```python
from build123d import *

# Parameters (mm, degrees)
SKETCH1_R           = 7.3
SKETCH1_R_2         = 2.4
BOSS_EXTRUDE1_DEPTH = 10
SKETCH2_R           = 8.8
SKETCH2_R_2         = 7.3
BOSS_EXTRUDE2_DEPTH = 3
SKETCH3_R           = 8.8
SKETCH3_R_2         = 2.4
BOSS_EXTRUDE3_DEPTH = 6
SKETCH4_R           = 4.2
SKETCH4_R_2         = 2.4
CUT_EXTRUDE1_DEPTH  = 43
BOSS_EXTRUDE4_REACH = 18
SKETCH5_R           = 7.5
SKETCH5_R_2         = 7.3
SKETCH6_R           = 4.2
SKETCH6_R_2         = 4.1
BOSS_EXTRUDE5_DEPTH = 16


with BuildPart() as part:
    # Sketch1 → Boss-Extrude1 (new body)
    with BuildSketch(Plane(origin=(0, 0, 0), x_dir=(1, 0, 0), z_dir=(0, 1, 0))):
        Circle(SKETCH1_R)
        Circle(SKETCH1_R_2, mode=Mode.SUBTRACT)
    extrude(amount=BOSS_EXTRUDE1_DEPTH)

    # Sketch2 → Boss-Extrude2 (add)
    with BuildSketch(Plane(origin=(0, 10, 0), x_dir=(1, 0, 0), z_dir=(0, 1, 0))):
        Circle(SKETCH2_R)
        Circle(SKETCH2_R_2, mode=Mode.SUBTRACT)
    extrude(amount=-BOSS_EXTRUDE2_DEPTH)

    # Sketch3 → Boss-Extrude3 (add)
    with BuildSketch(Plane(origin=(0, 10, 0), x_dir=(1, 0, 0), z_dir=(0, 1, 0))):
        Circle(SKETCH3_R)
        Circle(SKETCH3_R_2, mode=Mode.SUBTRACT)
    extrude(amount=BOSS_EXTRUDE3_DEPTH)

    # Sketch4 → Cut-Extrude1 (cut)
    with BuildSketch(Plane(origin=(0, 16, 0), x_dir=(1, 0, 0), z_dir=(0, 1, 0))):
        Circle(SKETCH4_R)
        Circle(SKETCH4_R_2, mode=Mode.SUBTRACT)
    extrude(amount=-CUT_EXTRUDE1_DEPTH, mode=Mode.SUBTRACT)

    # Sketch5 → Boss-Extrude4 (add, up to next)
    with BuildSketch(Plane.XZ, mode=Mode.PRIVATE) as boss_extrude4_sk1:
        Circle(SKETCH5_R)
        Circle(SKETCH5_R_2, mode=Mode.SUBTRACT)
    boss_extrude4_tool1 = extrude(boss_extrude4_sk1.sketch, amount=-BOSS_EXTRUDE4_REACH, mode=Mode.PRIVATE) - part.part
    add(boss_extrude4_tool1.solids().sort_by_distance((-7.478787, 0, 0))[0])

    # Sketch6 → Boss-Extrude5 (add)
    with BuildSketch(Plane.XZ):
        Circle(SKETCH6_R)
        Circle(SKETCH6_R_2, mode=Mode.SUBTRACT)
    extrude(amount=-BOSS_EXTRUDE5_DEPTH)


solid = part.part
```
The listing builds one solid part. Answer for the finished solid, in the listing's coordinates (mm). Give positions to 0.01 mm unless a question says otherwise; leave off trailing zeros. Order: outer loops, then holes, each group sorted by start corner. A loop starts at its lowest first (then second) coordinate and runs counter-clockwise, first axis right, second up. Notation, with made-up numbers: (54, -32) -> (69, -32) arc R26 cw to (69, 0) -> close; hole circle Ø5 at (67, -5). An arc over 180 degrees is marked (long way). One line per item, written item: value.
1) Find section C-C, the plane y = 4.25. Determine the outline of the cut face in (x, z), plus the area to 3 significant figures.
Reported:
outline: circle Ø15 at (0, 0); hole circle Ø8.2 at (0, 0)
area: 124 mm^2
2) Find section D-D, the plane z = -6.5. Determine the outline of the cut face in (x, y), plus the area to 3 significant figures.
Reported:
outline: (-5.93, 7) -> (-3.74, 7) -> (-3.74, 0) -> (3.74, 0) -> (3.74, 7) -> (5.93, 7) -> (5.93, 16) -> (-5.93, 16) -> close
area: 159 mm^2
3) Find the intervals of material crossed by line 1 (Z direction, x = 0, y = 9.25); line 2 (Z direction, x = -1.75, y = 8.5); line 3 (X direction, y = 6.75, z = -1.25), in increasing order.
Reported:
line 1: z = -8.8 to -4.1, 4.1 to 8.8
line 2: z = -8.62 to -3.71, 3.71 to 8.62
line 3: x = -7.4 to -3.9, 3.9 to 7.4
4) Determine the mould class of faces 1 (the flat face through (-4, 7, -7)), 2 (the cylindrical face through (-7.493, 3.451, 0.33)), 3 (the cylindrical face through (-0.534, 7.888, 4.065)) for opening direction Z: pulls with the +Z half, pulls with the -Z half, needs draft (parallel to the pull), parting line crosses it, or undercut.
Reported:
face 1: needs draft
face 2: parting line crosses it
face 3: undercut
5) Find section B-B, the plane x = 0. Determine the outline of the cut face in (y, z), plus the area to 3 significant figures.
Reported:
outline: (0, -7.5) -> (7, -7.5) -> (7, -8.8) -> (16, -8.8) -> (16, -4.1) -> (0, -4.1) -> close; (0, 4.1) -> (16, 4.1) -> (16, 8.8) -> (7, 8.8) -> (7, 7.5) -> (0, 7.5) -> close
area: 132 mm^2
6) A flat-ended cylindrical pin translates along its axis: P1, Ø1.5, axis at x = -4.5, y = 9.5, coming from the -Z side. Find the tip coordinate at first contact, or state that the pin passes through.
Reported:
P1: stops at z = -7.96
7) Find section A-A, the plane z = 0. Determine the outline of the cut face in (x, y).
Reported:
outline: (-8.8, 7) -> (-7.5, 7) -> (-7.5, 0) -> (-4.1, 0) -> (-4.1, 16) -> (-8.8, 16) -> close; (4.1, 0) -> (7.5, 0) -> (7.5, 7) -> (8.8, 7) -> (8.8, 16) -> (4.1, 16) -> close
